Work out the finished part from the listing and answer in its coordinate system (mm). Coordinates: 2 decimals unless noted, no trailing zeros. Order: outer loops, then holes, each group sorted by start corner. A loop starts at its lowest first (then second) coordinate and runs counter-clockwise, first axis right, second up. Notation, with made-up numbers: M 76.5,41 L 99.5,41 A25 ccw 99.5,71 Z; hole C 45.25,17 d5. An arc over 180 degrees is marked long. Use a Markdown table: item, result. Add a question column.
from build123d import *

# Parameters (mm, degrees)
CYLINDER1296_R               = 1.5
CYLINDER1296_DEPTH           = 12
CYLINDER1296_PLACEMENT_ANGLE = 45
CYLINDER1297_R               = 1.5
CYLINDER1297_DEPTH           = 12
CYLINDER1301_R               = 1.5
CYLINDER1301_DEPTH           = 12
CYLINDER1301_PLACEMENT_ANGLE = 135
CYLINDER1300_R               = 1.5
CYLINDER1300_DEPTH           = 12
CYLINDER1302_R               = 1.5
CYLINDER1302_DEPTH           = 12
CYLINDER1302_PLACEMENT_ANGLE = 225
CYLINDER1299_R               = 1.5
CYLINDER1299_DEPTH           = 12
CYLINDER1295_R               = 1.5
CYLINDER1295_DEPTH           = 12
CYLINDER1295_PLACEMENT_ANGLE = 45
CYLINDER1298_R               = 1.5
CYLINDER1298_DEPTH           = 12
COMPOUND928_PLACEMENT_ANGLE  = 22.5
TUBE114_R                    = 46
TUBE114_R_2                  = 36
TUBE114_DEPTH                = 1


with BuildPart() as obj1:
    # Cylinder1296 → Cylinder1296 (new body)
    with BuildSketch(Plane.XY):
        Circle(CYLINDER1296_R)
    extrude(amount=CYLINDER1296_DEPTH)


with BuildPart() as obj1_1:
    # Cylinder1296 placement: moved
    add(obj1.part.moved(Location((29.698485, -29.698485, 33.5))).rotate(Axis((29.698485, -29.698485, 33.5), (0, 0, 1)), CYLINDER1296_PLACEMENT_ANGLE))


with BuildPart() as obj2:
    # Cylinder1297 → Cylinder1297 (new body)
    with BuildSketch(Plane(origin=(42, 0, 33.5), x_dir=(0, 1, 0), z_dir=(0, 0, 1))):
        Circle(CYLINDER1297_R)
    extrude(amount=CYLINDER1297_DEPTH)


with BuildPart() as obj3:
    # Cylinder1301 → Cylinder1301 (new body)
    with BuildSketch(Plane.XY):
        Circle(CYLINDER1301_R)
    extrude(amount=CYLINDER1301_DEPTH)


with BuildPart() as obj3_1:
    # Cylinder1301 placement: moved
    add(obj3.part.moved(Location((29.698485, 29.698485, 33.5))).rotate(Axis((29.698485, 29.698485, 33.5), (0, 0, 1)), CYLINDER1301_PLACEMENT_ANGLE))


with BuildPart() as obj4:
    # Cylinder1300 → Cylinder1300 (new body)
    with BuildSketch(Plane(origin=(0, 42, 33.5), x_dir=(-1, 0, 0), z_dir=(0, 0, 1))):
        Circle(CYLINDER1300_R)
    extrude(amount=CYLINDER1300_DEPTH)


with BuildPart() as obj5:
    # Cylinder1302 → Cylinder1302 (new body)
    with BuildSketch(Plane.XY):
        Circle(CYLINDER1302_R)
    extrude(amount=CYLINDER1302_DEPTH)


with BuildPart() as obj5_1:
    # Cylinder1302 placement: moved
    add(obj5.part.moved(Location((-29.698485, 29.698485, 33.5))).rotate(Axis((-29.698485, 29.698485, 33.5), (0, 0, 1)), CYLINDER1302_PLACEMENT_ANGLE))


with BuildPart() as obj6:
    # Cylinder1299 → Cylinder1299 (new body)
    with BuildSketch(Plane(origin=(-42, 0, 33.5), x_dir=(0, -1, 0), z_dir=(0, 0, 1))):
        Circle(CYLINDER1299_R)
    extrude(amount=CYLINDER1299_DEPTH)


with BuildPart() as obj7:
    # Cylinder1295 → Cylinder1295 (new body)
    with BuildSketch(Plane.XY):
        Circle(CYLINDER1295_R)
    extrude(amount=CYLINDER1295_DEPTH)


with BuildPart() as obj7_1:
    # Cylinder1295 placement: moved
    add(obj7.part.moved(Location((-29.698485, -29.698485, 33.5))).rotate(Axis((-29.698485, -29.698485, 33.5), (0, 0, -1)), CYLINDER1295_PLACEMENT_ANGLE))


with BuildPart() as compound928:
    # Cylinder1298 → Cylinder1298 (new body)
    with BuildSketch(Plane(origin=(0, -42, 33.5), x_dir=(1, 0, 0), z_dir=(0, 0, 1))):
        Circle(CYLINDER1298_R)
    extrude(amount=CYLINDER1298_DEPTH)

    # Compound928: union obj1, obj2, obj3, obj4, obj5, obj6, obj7
    add(obj1_1.part)
    add(obj2.part)
    add(obj3_1.part)
    add(obj4.part)
    add(obj5_1.part)
    add(obj6.part)
    add(obj7_1.part)


with BuildPart() as compound928_1:
    # Compound928 placement: moved
    add(compound928.part.moved(Location((0, 0, 4))).rotate(Axis((0, 0, 4), (0, 0, 1)), COMPOUND928_PLACEMENT_ANGLE))


with BuildPart() as j_midi_deep_thin_actuator_washer:
    # Tube114 → Tube114 (new body)
    with BuildSketch(Plane.XY.offset(45)):
        Circle(TUBE114_R)
        Circle(TUBE114_R_2, mode=Mode.SUBTRACT)
    extrude(amount=TUBE114_DEPTH)

    # Cut469: cut Compound928
    add(compound928_1.part, mode=Mode.SUBTRACT)


with BuildPart() as j_midi_deep_thin_actuator_washer_1:
    # Cut469 placement: moved
    add(j_midi_deep_thin_actuator_washer.part.moved(Location((0, 0, 4))))


solid = j_midi_deep_thin_actuator_washer_1.part
(1) The mould has two halves that part along Y. Classify faces 1 (the flat face through (23.6, 27.5, 49)), 2 (the cylindrical face through (14.844, 37.943, 49.493)), 3 (the cylindrical face through (-5.99, 45.61, 49.49)): pulls with the +Y half, pulls with the -Y half, needs draft (parallel to the pull), parting line crosses it, or undercut.
(2) A cutting plane is placed at C-C on z = 49.4. Count the separate pieces of the cut face and the enclosed holes in it, plus the area to 3 significant figures.
(3) A cutting plane is placed at A-A on x = 0. Write down the section's boundary in (y, z).
(4) Given P1, Ø4, axis at x = 38.8, y = -16.07, coming from the +Z side, flat-ended and moving along its own axis, determine where the tip first touches the part or whether it passes through.
(5) Straight lines are drawn through the part: line 1 (X direction, y = 38, z = 49.4); line 2 (Y direction, x = -20, z = 49.8); line 3 (Y direction, x = 40, z = 49.15). For each, find the intervals that lie inside material, in ascending order.
From the geometry:
| question | item | result |
|---|---|---|
| 1 | face 1 | needs draft |
| 1 | face 2 | undercut |
| 1 | face 3 | parting line crosses it |
| 2 | separate pieces | 1 |
| 2 | enclosed holes | 9 |
| 2 | area | 2,520 mm2 |
| 3 | outline | M -46,49 L -36,49 L -36,50 L -46,50 Z; M 36,49 L 46,49 L 46,50 L 36,50 Z |
| 4 | P1 | stops at z = 50 |
| 5 | line 1 | x = -25.92 to -17.34, -14.81 to 14.81, 17.34 to 25.92 |
| 5 | line 2 | y = -41.42 to -29.93, 29.93 to 41.42 |
| 5 | line 3 | y = -22.72 to -16.98, -15.17 to 15.17, 16.98 to 22.72 |
